```python
from build123d import *

# Parameters (mm, degrees)
EXTRUDE_1_DEPTH     = 220
CUT_EXTRUDE_1_DEPTH = 26


with BuildPart() as part:
    # Эскиз1 → Вытянуть-Тонкостенный1 (new body)
    with BuildSketch(Plane(origin=(0, 0, 0), x_dir=(0, 0, -1), z_dir=(1, 0, 0))):
        Polygon((0, 25), (0, 0), (25, 0), (25, 2), (2, 2), (2, 25), align=None)
    extrude(amount=EXTRUDE_1_DEPTH)

    # Эскиз3 → Вырез-Вытянуть1 (cut, through all)
    with BuildSketch(Plane.XZ):
        Polygon((0, -25), (14.444982857, -18.190263819), (31.898443386, -25), align=None)
        Polygon((40, -25), (54.444982857, -18.190263819), (71.898443386, -25), align=None)
        Polygon((80, -25), (94.444982857, -18.190263819), (111.898443386, -25), align=None)
        Polygon((120, -25), (134.444982857, -18.190263819), (151.898443386, -25), align=None)
        Polygon((160, -25), (174.444982857, -18.190263819), (191.898443386, -25), align=None)
    extrude(amount=-CUT_EXTRUDE_1_DEPTH, mode=Mode.SUBTRACT)


solid = part.part
```
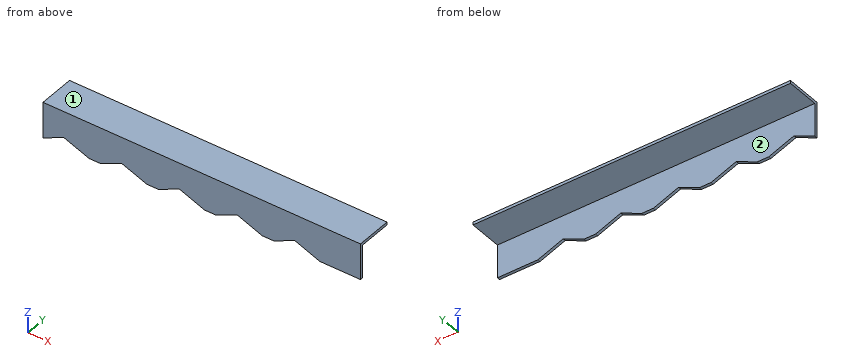
Verification items for the finished model (mm, model axes). Face numbers are marked on the shaded views. A direction names the side the tool comes from. Coordinates: 2 decimals unless noted, no trailing zeros. Loops run counter-clockwise (first coordinate to the right, second up) from the corner with the lowest first, then second, coordinate; pieces in that order, holes last. Notation, with made-up numbers: (65.5, 3) -> (118.5, 3) arc R19 cw to (118.5, 31) -> close; hole circle Ø10 at (-35.5, 51.25). An arc over 180 degrees is marked (long way). Answer in a Markdown table with one row per item. Add a question column.
1. Access from +Z, -Z, +X, -X, +Y, -Y to the whole of each face (thin tool, end or side, straight path). Record for the marked faces 1 and 2.
2. Section check A-A, the plane z = -20.5. Enter the section's corners in (x, y), then the cut area to 3 significant figures.
3. Section check B-B, the plane x = 184.5. Enter the section's corners in (y, z), then the cut area to 3 significant figures.
4. Section check C-C, the plane y = 6. Enter the section's corners in (x, z).
5. Depth check by flat-ended pin: P1, Ø1, axis at x = 50, y = 12, coming from the -Z side; P2, Ø4, axis at x = 134, z = -7, coming from the +Y side; P3, Ø10, axis at y = 3.5, z = -11.5, coming from the -X side. Enter the tip coordinate at first touch or a pass-through.
6. Section check D-D, the plane z = -9.75. Enter the section's corners in (x, y), then the cut area to 3 significant figures.
7. Material ranges on probe 1 along Y at (x, z) = (54, -16.75); probe 2 along Z at (x, y) = (165, 10.75), recorded low to high. Write a range as [from, to].
Derived:
| question | item | result |
|---|---|---|
| 1 | face 1 | +Z, +X, -X, +Y, -Y |
| 1 | face 2 | -Z, +X, -X, +Y |
| 2 | outline | (0, 0) -> (9.55, 0) -> (9.55, 2) -> (0, 2) -> close; (20.36, 0) -> (49.55, 0) -> (49.55, 2) -> (20.36, 2) -> close; (60.36, 0) -> (89.55, 0) -> (89.55, 2) -> (60.36, 2) -> close; (100.36, 0) -> (129.55, 0) -> (129.55, 2) -> (100.36, 2) -> close; (140.36, 0) -> (169.55, 0) -> (169.55, 2) -> (140.36, 2) -> close; (180.36, 0) -> (220, 0) -> (220, 2) -> (180.36, 2) -> close |
| 2 | area | 332 mm² |
| 3 | outline | (0, -22.11) -> (2, -22.11) -> (2, -2) -> (25, -2) -> (25, 0) -> (0, 0) -> close |
| 3 | area | 90.2 mm² |
| 4 | outline | (0, -2) -> (220, -2) -> (220, 0) -> (0, 0) -> close |
| 5 | P1 | stops at z = -2 |
| 5 | P2 | stops at y = 2 |
| 5 | P3 | stops at x = 0 |
| 6 | outline | (0, 0) -> (220, 0) -> (220, 2) -> (0, 2) -> close |
| 6 | area | 440 mm² |
| 7 | probe 1 | y = [0, 2] |
| 7 | probe 2 | z = [-2, 0] |
